Job drawing, mm, ordinate dimensions from the low corner. One solid piece. Coordinates: 2 decimals unless noted, no trailing zeros. Write each loop counter-clockwise with the first axis right and the second up, starting at its lowest first coordinate (ties: lowest second). Pieces come first, ordered by that corner, then holes. Notation, with made-up numbers: (46.5, 0.25) - (81.5, 0.25) arc R15 ccw to (81.5, 25.25) - close; hole circle Ø11 at (16.5, 1.25). An arc over 180 degrees is marked (long way). Put each result on its own line as item: value. Start each with the question number.
1. Drill centre lines: L1, parallel to Y at x = 6, z = 3.8; L2, parallel to Z at x = 5.75, y = 5.25; L3, parallel to Y at x = 5, z = 3.9. Where is each one in solid material? Low to high. Write a range as from..to.
2. Saw through at B-B, the plane y = 5.75. Write the cut outline in (x, z), plus the area to 3 significant figures.
3. Saw through at A-A, the plane x = 2.5. Write the cut outline in (y, z).
4. Saw through at C-C, the plane z = 4.55. Write the cut outline in (x, y), plus the area to 3 significant figures.
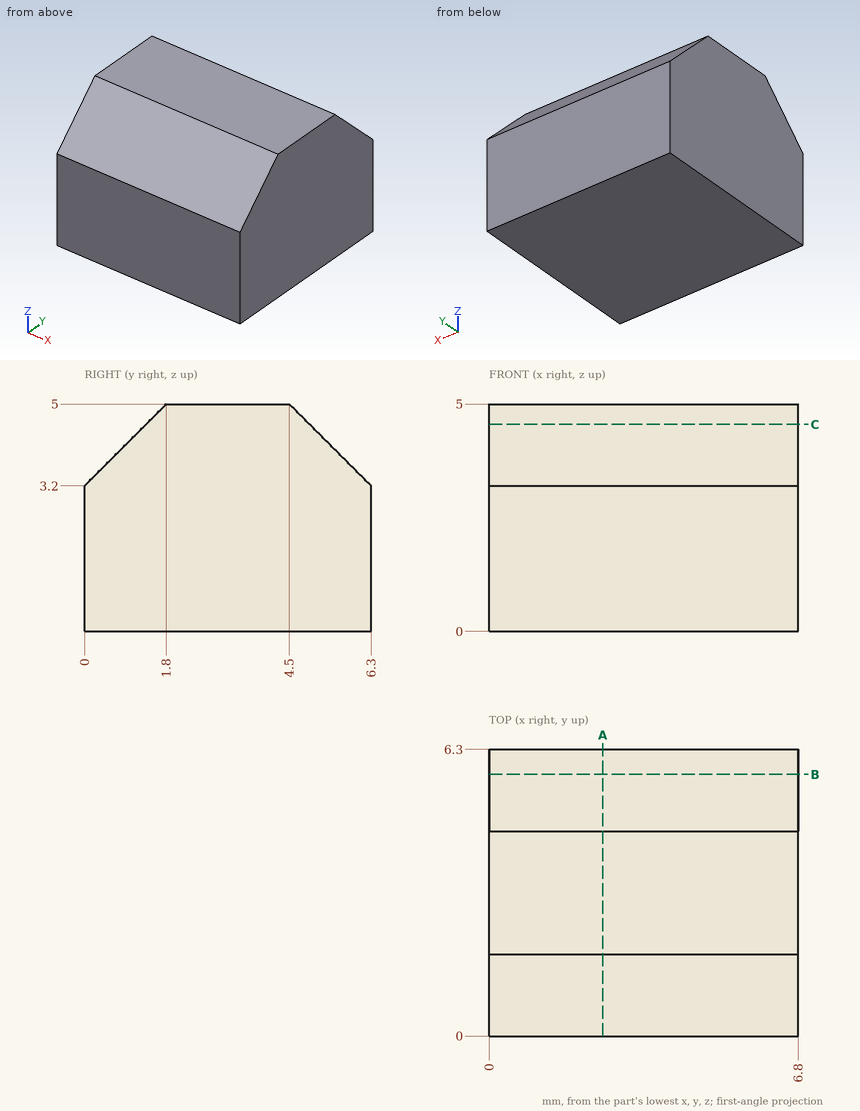
Final values:
1. L1: y = 0.6..5.7
1. L2: z = 0..4.25
1. L3: y = 0.7..5.6
2. outline: (0, 0) - (6.8, 0) - (6.8, 3.75) - (0, 3.75) - close
2. area: 25.5 mm²
3. outline: (0, 0) - (6.3, 0) - (6.3, 3.2) - (4.5, 5) - (1.8, 5) - (0, 3.2) - close
4. outline: (0, 1.35) - (6.8, 1.35) - (6.8, 4.95) - (0, 4.95) - close
4. area: 24.5 mm²
